The listing builds one solid part. Answer for the finished solid, in the listing's coordinates (mm). A direction names the side the tool comes from. Coordinates: 2 decimals unless noted, no trailing zeros. Write each loop counter-clockwise with the first axis right and the second up, starting at its lowest first coordinate (ties: lowest second). Pieces come first, ordered by that corner, then holes.
Autodesk Inventor part; units mm, degrees
ref_plane "作業平面1" through (0, 0, 14) normal (0, 0, 1) x (-0.9659258, -0.258819, 0)
ref_plane "YZ Plane" through (0, 0, 0) normal (1, 0, 0) x (0, 1, 0)
ref_plane "XZ Plane" through (0, 0, 0) normal (0, 1, 0) x (-1, 0, 0)
ref_plane "作業平面1" through (0, 0, 14) normal (0, 0, 1) x (-0.9659258, -0.258819, 0)
sketch "スケッチ14" plane through (0, 0, 0) normal (0, 0, 1) x (1, 0, 0)
  circle A0 centre (0, 0) radius 25
  circle A1 centre (30, 0) radius 4.025
  line L0 (0, 25) -> (40, 25)
  line L1 (40, 25) -> (40, -25)
  line L2 (40, -25) -> (0, -25)
  line L3 (0, -25) -> (0, 25)
  line L4 (0, -25) -> (40, -10.4412)
  line L5 (0, 25) -> (40, 10.4412)
  line L6 (0.5157, 26.4168) -> (40.5157, 11.858)
  line L7 (0.5157, -26.4168) -> (40.5157, -11.858)
  circle A2 centre (0, 0) radius 6.5
  line L8 (40.5157, -11.858) -> (63.847, -3.366)
  line L9 (37.8689, 40.3876) -> (23.4147, 35.1267)
  line L10 (23.4147, 35.1267) -> (-16.5853, 20.5679)
  line L11 (-16.5853, 20.5679) -> (-32.0428, 14.9418)
  line L12 (-32.0428, 14.9418) -> (-14.9418, -32.0428)
  line L13 (-14.9418, -32.0428) -> (0.5157, -26.4168)
  line L14 (40, 12.0456) -> (47.7428, -9.2275)
  line L15 (40, 12.0456) -> (30.6418, 37.7571)
  point P0 (8.5505, -23.4923)
  point P1 (40, -12.0456)
  point P2 (40, 12.0456)
  point P3 (8.5505, 23.4923)
  dimension "d111" = 50
  dimension "d112" = 8.05
  dimension "d113" = 30
  dimension "d114" = 40
  dimension "d115" = 50
  dimension "d116" = 25
  dimension "d119" = 25
  dimension "d126" = 20
  dimension "d127" = 20
  dimension "d144" = 13
  dimension "d201" = 90
  dimension "d202" = 90
extrude "押し出し9" add sketch "スケッチ14" along normal blind 5 contours A0 L4 L3 A2 L5 | A0 L5 L1 L4 | L5 A0 | A0 L6 L1 L5 | L4 L1 L7 A0 | A0 L4 | L3 A2 A0
sketch "スケッチ15" plane through (0, 0, 0) normal (0, 0, -1) x (-1, 0, 0)
  circle A0 centre (-30, 0) radius 4.025
  circle A1 centre (-30, 0) radius 6.6
  line L0 (-24.4, 3.4928) -> (-24.4, -3.4928)
  arc A2 (-24.4, 1.4928) -> (-24.4, 3.4928) centre (-24.4, 2.4928) ccw
  arc A3 (-24.4, -3.4928) -> (-24.4, -1.4928) centre (-24.4, -2.4928) ccw
  point P0 (0, 0)
  dimension "d122" = 13.2
  dimension "d203" = 5.6
  dimension "d204" = 1
  dimension "d205" = 1
  dimension "d206" = 0
  dimension "d207" = 0
extrude "押し出し10" cut sketch "スケッチ15" against normal blind 2 contours L0 A1 | A2 A1 | A1 A2 L0 | L0 A3 A1 | A1 A3
sketch "スケッチ16" plane through (0, 0, 5) normal (0, 0, 1) x (1, 0, 0)
  circle A0 centre (30, 0) radius 4.025
  circle A1 centre (30, 0) radius 17
  arc A2 (8.5505, 23.4923) -> (8.5505, -23.4923) centre (0, 0) ccw
  circle A3 centre (0, 0) radius 25
  line L0 (40, -12.0456) -> (40, 12.0456)
  line L1 (40, 12.0456) -> (-0.2187, 26.6841)
  line L2 (40, -12.0456) -> (-2.6962, -27.5858)
  circle A4 centre (0, 0) radius 17.5
  line L3 (8.5505, 23.4923) -> (5.9854, 16.4446)
  line L4 (-17.5, 0) -> (-25, 0)
  line L5 (-2.7839, 19.6364) -> (32.5, 6.7941)
  line L6 (32.5, 6.7941) -> (32.5, -6.7941)
  line L7 (32.5, -6.7941) -> (-5.2613, -20.5381)
  line L8 (17.9474, 20.0721) -> (15.3823, 13.0244)
  line L9 (-17.5, 0) -> (0, 0)
  line L10 (-13.6656, -12.9367) -> (-0.4151, -19.1155)
  line L11 (-7.0404, -16.0261) -> (-11.4484, -25.4792)
  line L12 (17.2336, 18.1109) -> (11.4362, 13.2463)
  line L13 (18.0185, 5.7516) -> (7.3857, 18.4233)
  line L14 (0, 25) -> (0, 10.5586)
  line L15 (17.2336, 18.1109) -> (19.0798, 19.66)
  point P0 (0, -25)
  point P1 (-11.8057, -12.918)
  point P2 (-10.2087, -22.8207)
  point P3 (-7.3958, -15.8604)
  dimension "d125" = 34
  dimension "d128" = 7.5
  dimension "d164" = 7.5
  dimension "d165" = 10
  dimension "d186" = 90
  dimension "d187" = 65
  dimension "d196" = 30
extrude "押し出し11" add sketch "スケッチ16" along normal blind 12 contours L12 L5 L3 A3 | A3 L1 L8 | L8 L1 L15 | L3 L5 L14 A2 | L12 L13 L5 | A2 L4 A4 L10 L11 | L14 A4 L4 A2 | L5 L13 L12 A4 | A4 L14 L5
sketch "スケッチ17" plane through (0, 0, 5) normal (0, 0, 1) x (1, 0, 0)
  circle A0 centre (30, 0) radius 4.025
  line L0 (0, 0) -> (30, 0)
  circle A1 centre (0, 0) radius 12.5
  line L1 (0, 0) -> (12.4415, 7.1831)
  point P0 (10.8253, 6.25)
  point P1 (0, 12.5)
  point P2 (-10.8253, 6.25)
  point P3 (-10.8253, -6.25)
  point P4 (0, -12.5)
  point P5 (10.8253, -6.25)
  dimension "d131" = 25
  dimension "d132" = 30
  dimension "d135" = 360
hole "穴5" at (10.8253, 6.25, 5) at (0, 12.5, 5) at (-10.8253, 6.25, 5) at (-10.8253, -6.25, 5) at (0, -12.5, 5) at (10.8253, -6.25, 5) direction (0, 0, -1) diameter 3.2 end through all
sketch "スケッチ18" plane through (0, 0, 5) normal (0, 0, 1) x (1, 0, 0)
  circle A0 centre (30, 0) radius 4.025
  line L0 (0, 0) -> (30, 0)
  circle A1 centre (0, 0) radius 10.2
  point P0 (10.2, 0)
  point P1 (-5.1, 8.8335)
  point P2 (-5.1, -8.8335)
  dimension "d145" = 20.4
  dimension "d148" = 360
hole "穴6" at (10.2, 0, 5) at (-5.1, 8.8335, 5) at (-5.1, -8.8335, 5) direction (0, 0, -1) diameter 4.2 end through all
sketch "スケッチ19" plane through (0, 0, 5) normal (0, 0, 1) x (1, 0, 0)
  circle A0 centre (0, 12.5) radius 1.6
  circle A1 centre (0, 0) radius 12.5
  circle A2 centre (0, 12.5) radius 3
  circle A3 centre (-10.8253, 6.25) radius 3
  circle A4 centre (-10.8253, -6.25) radius 3
  circle A5 centre (0, -12.5) radius 3
  circle A6 centre (10.8253, -6.25) radius 3
  circle A7 centre (10.8253, 6.25) radius 3
  dimension "d157" = 6
  dimension "d160" = 360
extrude "押し出し12" cut sketch "スケッチ19" against normal blind 3 contours A0 A1 | A0 A1 A2 | A1 A0 | A0 A1 A2 | A3 A1 | A1 A3 | A7 A1 | A1 A7 | A4 A1 | A1 A4 | A6 A1 | A1 A6 | A5 A1 | A1 A5
sketch "スケッチ20" plane through (0, 0, 17) normal (0, 0, 1) x (1, 0, 0)
  line L0 (19.0798, 19.66) -> (8.5505, 23.4923)
  line L1 (17.9474, 20.0721) -> (15.3823, 13.0244)
  line L2 (15.3823, 13.0244) -> (5.9854, 16.4446)
  line L3 (5.9854, 16.4446) -> (8.5505, 23.4923)
  line L4 (0, 0) -> (0, 30.7788)
  circle A0 centre (0, 0) radius 21.25
  circle A1 centre (0, 0) radius 25
  point P0 (11.9664, 18.2584)
  point P1 (0, 21.25)
  point P2 (-10.625, 18.403)
  point P3 (-18.403, 10.625)
  point P4 (-21.25, 0)
  point P5 (-18.403, -10.625)
  point P6 (-10.625, -18.403)
  point P7 (0, -21.25)
  point P8 (10.625, -18.403)
  point P9 (18.403, -10.625)
  point P10 (21.25, 0)
  point P11 (18.403, 10.625)
  point P12 (10.625, 18.403)
  dimension "d167" = 7.5
  dimension "d168" = 5
  dimension "d169" = 3.75
  dimension "d170" = 3.75
  dimension "d171" = 50
  dimension "d174" = 360
hole "穴7" at (10.625, 18.403, 17) at (0, 21.25, 17) at (-10.625, 18.403, 17) at (-18.403, 10.625, 17) direction (0, 0, -1) diameter 2.459 depth 10
fillet "フィレット9" radius 17 2 edges at (40, 12.0456, 2.5) (40, -12.0456, 2.5)
sketch "スケッチ21" plane through (0, 0, 17) normal (0, 0, 1) x (1, 0, 0)
  circle A0 centre (-18.403, 10.625) radius 1.2295
  circle A1 centre (0, 0) radius 21.25
  line L0 (0, 0) -> (-31.1052, 0)
  point P0 (-21.25, 0)
  point P1 (-18.403, -10.625)
hole "穴8" at (-21.25, 0, 17) at (-18.403, -10.625, 17) direction (0, 0, -1) diameter 2.459 depth 10
fillet "フィレット12" radius 3.75 4 edges at (-7.0404, -16.0261, 11) (-10.2087, -22.8207, 11) (19.0798, 19.66, 11) (11.4362, 13.2463, 11)
properties part number "RP_Thigh-Base" material "アルミニウム 6061"
1. For a pull along X with two mould halves and no side action, classify faces 5 (the cylindrical face through (12.245, -6.988, 0.986)), 6 (the cylindrical face through (15.377, 19.063, 10.916)) as pulls with the +X half, pulls with the -X half, needs draft (parallel to the pull), parting line crosses it, or undercut.
Results found:
face 5: undercut
face 6: pulls with the +X half
2. Find the intervals of material crossed by L1, parallel to Y at x = -18, z = 12.5; L2, parallel to X at y = 0, z = 1.1; L3, parallel to X at y = 0, z = 15, in increasing order.
Results found:
L1: y = -17.35 to -11.79, -9.46 to 9.46, 11.79 to 17.35
L2: x = -25 to -6.5, 6.5 to 8.1, 12.3 to 24.4, 36.6 to 40
L3: x = -25 to -22.48, -20.02 to -17.5
3. Flat-ended cylindrical pins translate along their axes: P1, Ø6, axis at x = 27.5, y = -8, coming from the +Z side; P2, Ø5, axis at x = -10.83, y = 6.25, coming from the +Z side. Find the tip coordinate at first contact, or state that the pin passes through.
Results found:
P1: stops at z = 5
P2: stops at z = 2
4. A tool of negligible diameter and unlimited length cuts with its end or side. For faces 1 (the cylindrical face through (11.57, 14.27, 10.92)), 2 (the cylindrical face through (13.687, -5.349, 3.521)), 3 (the cylindrical face through (-8.307, -16.563, 10.916)), 4 (the cylindrical face through (-0.07, 14.1, 0.99)), from which of +Z, -Z, +X, -X, +Y, -Y can it reach the whole face along a straight path? Write none if from no direction.
Results found:
face 1: +Z, -Y
face 2: +Z
face 3: +Z, +X
face 4: +Z, -Z
5. Section B-B on x = 28 is taken. Give the vertices of the cut face in (y, z), then the cut area to 3 significant figures.
Results found:
outline: (-16.41, 0) - (-6.29, 0) - (-6.29, 2) - (-3.49, 2) - (-3.49, 5) - (-16.41, 5) - close; (3.49, 2) - (6.29, 2) - (6.29, 0) - (16.41, 0) - (16.41, 5) - (3.49, 5) - close
area: 118 mm2
6. Section A-A on x = 0 is taken. State how many separate pieces and enclosed holes the cut face has, then the cut area to 3 significant figures.
Results found:
separate pieces: 4
enclosed holes: 0
area: 202 mm2
